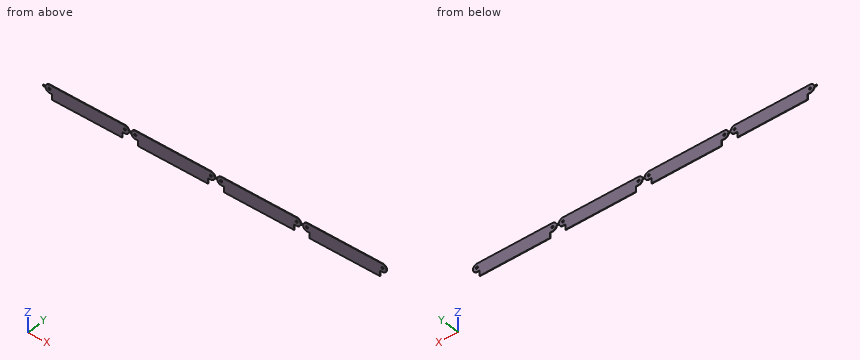
```python
from build123d import *

# Parameters (mm, degrees)
SKETCH1_R           = 2
BOSS_EXTRUDE1_DEPTH = 1


with BuildPart() as part:
    # Sketch1 → Boss-Extrude1 (new body)
    with BuildSketch(Plane(origin=(0, 0, 0), x_dir=(1, 0, 0), z_dir=(0, 1, 0))):
        with BuildLine():
            Line((5, 7.5), (0, 7.5))
            ThreePointArc((0, 7.5), (-4.937104415, 5.645794895), (-7.433034374, 1))
            Line((-7.433034374, 1), (-12.003034374, 1))
            Line((-12.003034374, 1), (-12.003034374, -1))
            Line((-12.003034374, -1), (-7.433034374, -1))
            ThreePointArc((-7.433034374, -1), (-4.937104415, -5.645794895), (0, -7.5))
            Line((0, -7.5), (142.5, -7.5))
            ThreePointArc((142.5, -7.5), (147.437104415, -5.645794895), (149.933034374, -1))
            Line((149.933034374, -1), (154.566965626, -1))
            ThreePointArc((154.566965626, -1), (157.062895585, -5.645794895), (162, -7.5))
            Line((162, -7.5), (304.5, -7.5))
            ThreePointArc((304.5, -7.5), (309.437104415, -5.645794895), (311.933034374, -1))
            Line((311.933034374, -1), (316.566965626, -1))
            ThreePointArc((316.566965626, -1), (319.062895585, -5.645794895), (324, -7.5))
            Line((324, -7.5), (466.5, -7.5))
            ThreePointArc((466.5, -7.5), (471.437104415, -5.645794895), (473.933034374, -1))
            Line((473.933034374, -1), (478.566965626, -1))
            ThreePointArc((478.566965626, -1), (481.062895585, -5.645794895), (486, -7.5))
            Line((486, -7.5), (628.5, -7.5))
            ThreePointArc((628.5, -7.5), (633.437104415, -5.645794895), (635.933034374, -1))
            Line((635.933034374, -1), (636, -1))
            Line((636, -1), (636, 1))
            Line((636, 1), (635.933034374, 1))
            ThreePointArc((635.933034374, 1), (633.437104415, 5.645794895), (628.5, 7.5))
            Line((628.5, 7.5), (623.5, 7.5))
            Line((623.5, 7.5), (623.5, 17.5))
            Line((623.5, 17.5), (491, 17.5))
            Line((491, 17.5), (491, 7.5))
            Line((491, 7.5), (486, 7.5))
            ThreePointArc((486, 7.5), (481.062895585, 5.645794895), (478.566965626, 1))
            Line((478.566965626, 1), (473.933034374, 1))
            ThreePointArc((473.933034374, 1), (471.437104415, 5.645794895), (466.5, 7.5))
            Line((466.5, 7.5), (461.5, 7.5))
            Line((461.5, 7.5), (461.5, 17.5))
            Line((461.5, 17.5), (329, 17.5))
            Line((329, 17.5), (329, 7.5))
            Line((329, 7.5), (324, 7.5))
            ThreePointArc((324, 7.5), (319.062895585, 5.645794895), (316.566965626, 1))
            Line((316.566965626, 1), (311.933034374, 1))
            ThreePointArc((311.933034374, 1), (309.437104415, 5.645794895), (304.5, 7.5))
            Line((304.5, 7.5), (299.5, 7.5))
            Line((299.5, 7.5), (299.5, 17.5))
            Line((299.5, 17.5), (167, 17.5))
            Line((167, 17.5), (167, 7.5))
            Line((167, 7.5), (162, 7.5))
            ThreePointArc((162, 7.5), (157.062895585, 5.645794895), (154.566965626, 1))
            Line((154.566965626, 1), (149.933034374, 1))
            ThreePointArc((149.933034374, 1), (147.437104415, 5.645794895), (142.5, 7.5))
            Line((142.5, 7.5), (137.5, 7.5))
            Line((137.5, 7.5), (137.5, 17.5))
            Line((137.5, 17.5), (5, 17.5))
            Line((5, 17.5), (5, 7.5))
        make_face()
        with Locations(Location((0, 0, 0), (0, 0, 270))):
            Circle(SKETCH1_R, mode=Mode.SUBTRACT)
        with Locations(Location((142.5, 0, 0), (0, 0, 270))):
            Circle(SKETCH1_R, mode=Mode.SUBTRACT)
        with Locations(Location((304.5, 0, 0), (0, 0, 270))):
            Circle(SKETCH1_R, mode=Mode.SUBTRACT)
        with Locations(Location((162, 0, 0), (0, 0, 270))):
            Circle(SKETCH1_R, mode=Mode.SUBTRACT)
        with Locations(Location((466.5, 0, 0), (0, 0, 270))):
            Circle(SKETCH1_R, mode=Mode.SUBTRACT)
        with Locations(Location((324, 0, 0), (0, 0, 270))):
            Circle(SKETCH1_R, mode=Mode.SUBTRACT)
        with Locations(Location((628.5, 0, 0), (0, 0, 270))):
            Circle(SKETCH1_R, mode=Mode.SUBTRACT)
        with Locations(Location((486, 0, 0), (0, 0, 270))):
            Circle(SKETCH1_R, mode=Mode.SUBTRACT)
    extrude(amount=BOSS_EXTRUDE1_DEPTH)


solid = part.part
```
For this review, take the finished solid that the model builds, in its own axes (mm). Coordinates: 2 decimals unless noted, no trailing zeros. Order: outer loops, then holes, each group sorted by start corner. A loop starts at its lowest first (then second) coordinate and runs counter-clockwise, first axis right, second up. Notation, with made-up numbers: (-15.5, 74) - (-11.5, 74) arc R23 ccw to (-11.5, 113) - close; hole circle Ø7 at (87, -17.5). An arc over 180 degrees is marked (long way). Answer as a JSON object with one key per item and string values. Group by question number.
1. We need section A-A on z = -13.5. State the section outline as (x, y) points, then the cut area to 3 significant figures.
2. We need section B-B on y = 0.3. Give the number of separate pieces and of enclosed holes in the cut face, then the cut area to 3 significant figures.
3. For probe 1 along X at (y, z) = (0.8, -14.25); probe 2 along Z at (x, y) = (466.5, 0.8); probe 3 along X at (y, z) = (0.5, 6.5), list the stretches that pass through material, from the lowest coordinate up.
4. Clearance check with flat-ended pins moving along their axes: P1, Ø0.5, axis at x = 314.5, y = 0.5, coming from the +Z side; P2, Ø5, axis at x = 139, z = 1, coming from the -Y side; P3, Ø2.5, axis at x = 324, z = 0, coming from the -Y side. State where each tip first meets the part, or that it passes through.
Final values:
{
 "1": {"outline": "(5, 0) - (137.5, 0) - (137.5, 1) - (5, 1) - close; (167, 0) - (299.5, 0) - (299.5, 1) - (167, 1) - close; (329, 0) - (461.5, 0) - (461.5, 1) - (329, 1) - close; (491, 0) - (623.5, 0) - (623.5, 1) - (491, 1) - close", "area": "530 mm²"},
 "2": {"separate pieces": "1", "enclosed holes": "8", "area": "14,500 mm²"},
 "3": {"probe 1": "5 to 137.5, 167 to 299.5, 329 to 461.5, 491 to 623.5", "probe 2": "-7.5 to -2, 2 to 7.5", "probe 3": "-3.74 to 146.24, 158.26 to 308.24, 320.26 to 470.24, 482.26 to 632.24"},
 "4": {"P1": "z = 1", "P2": "y = 0", "P3": "through"}
}
